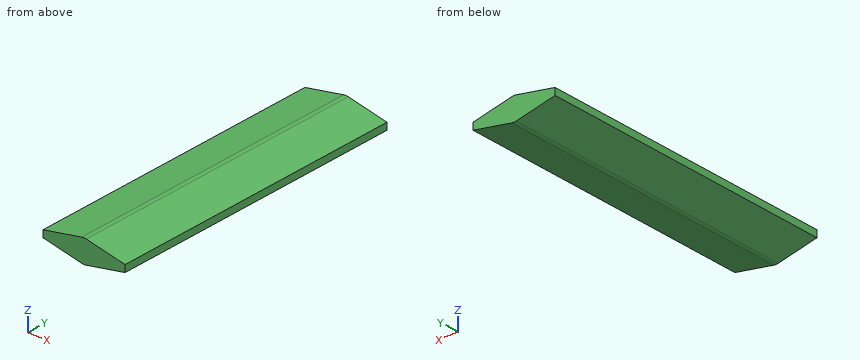
```python
from build123d import *

# Parameters (mm, degrees)
EXTRUDE_1_DEPTH = 650


with BuildPart() as part:
    # 草图5 → 凸台-拉伸1 (new body, symmetric)
    with BuildSketch(Plane(origin=(0, 0, 0), x_dir=(1, 0, 0), z_dir=(0, 1, 0))):
        with BuildLine():
            Line((180, 0), (180, -15.011157988))
            Line((180, -15.011157988), (9.8, -49.030194778))
            ThreePointArc((9.8, -49.030194778), (0, -50), (-9.8, -49.030194778))
            Line((-9.8, -49.030194778), (-180, -15.011157988))
            Line((-180, -15.011157988), (-180, 0))
            Line((-180, 0), (-180, 15.011157988))
            Line((-180, 15.011157988), (-9.799999967, 49.030194785))
            ThreePointArc((-9.799999967, 49.030194785), (1.7e-08, 50), (9.8, 49.030194778))
            Line((9.8, 49.030194778), (180, 15.011157988))
            Line((180, 15.011157988), (180, 0))
        make_face()
    extrude(amount=EXTRUDE_1_DEPTH, both=True)


solid = part.part
```
Verification items for the finished model (mm, model axes). Give positions to 0.01 mm unless a question says otherwise; leave off trailing zeros. Order: outer loops, then holes, each group sorted by start corner. A loop starts at its lowest first (then second) coordinate and runs counter-clockwise, first axis right, second up. Notation, with made-up numbers: (-15, 13) -> (29, 13) arc R19 ccw to (29, 45) -> close; hole circle Ø3 at (45.25, 77). An arc over 180 degrees is marked (long way). Use a Markdown table: item, result.
1) Section check B-B, the plane x = -61. Record the boundary of the cut face in (y, z).
Results:
| item | result |
|---|---|
| outline | (-650, -38.8) -> (650, -38.8) -> (650, 38.8) -> (-650, 38.8) -> close |
2) Material ranges on probe 1 along Z at (x, y) = (-73.5, 544); probe 2 along Z at (x, y) = (-15, 353), recorded low to high.
Results:
| item | result |
|---|---|
| probe 1 | -36.3 to 36.3 |
| probe 2 | -47.99 to 47.99 |
3) Section check C-C, the plane z = -38. Record the boundary of the cut face in (x, y).
Results:
| item | result |
|---|---|
| outline | (-64.98, -650) -> (64.98, -650) -> (64.98, 650) -> (-64.98, 650) -> close |
4) Depth check by flat-ended pin: pin 1 Ø3 at (x, y) = (-113.5, 256) entering from +Z; pin 2 Ø4 at (x, y) = (73, 271) entering from -Z. Enter the tip coordinate at first touch or a pass-through.
Results:
| item | result |
|---|---|
| pin 1 | z = 28.6 |
| pin 2 | z = -36.8 |
5) Section check A-A, the plane y = -444.5. Record the boundary of the cut face in (x, z), then the cut area to 3 significant figures.
Results:
| item | result |
|---|---|
| outline | (-180, -15.01) -> (-9.8, -49.03) arc R50 ccw to (9.8, -49.03) -> (180, -15.01) -> (180, 15.01) -> (9.8, 49.03) arc R50 ccw to (-9.8, 49.03) -> (-180, 15.01) -> close |
| area | 23,700 mm² |
